```python
from build123d import *

# Parameters (mm, degrees)
SKETCH1_W           = 38
SKETCH1_H           = 41.8
SKETCH1_W_2         = 34.6
SKETCH1_H_2         = 40
BOSS_EXTRUDE1_DEPTH = 100
SKETCH2_W           = 1.7
SKETCH2_H           = 25
BOSS_EXTRUDE2_DEPTH = 13.6
BOSS_EXTRUDE5_DEPTH = 25
SKETCH6_W           = 38
SKETCH6_H           = 41.8
BOSS_EXTRUDE6_DEPTH = 0.6
SKETCH7_W           = 13.3
SKETCH7_H           = 4.4
CUT_EXTRUDE1_DEPTH  = 10
CUT_EXTRUDE2_DEPTH  = 10


with BuildPart() as part:
    # Sketch1 → Boss-Extrude1 (new body)
    with BuildSketch(Plane(origin=(0, 0, 0), x_dir=(1, 0, 0), z_dir=(0, 1, 0))):
        Rectangle(SKETCH1_W, SKETCH1_H)
        Rectangle(SKETCH1_W_2, SKETCH1_H_2, mode=Mode.SUBTRACT)
    extrude(amount=BOSS_EXTRUDE1_DEPTH)

    # Sketch2 → Boss-Extrude2 (add)
    with BuildSketch(Plane(origin=(0, 100, 0), x_dir=(1, 0, 0), z_dir=(0, 1, 0))):
        with Locations((18.15, 0)):
            Rectangle(SKETCH2_W, SKETCH2_H)
        with Locations((-18.15, 0)):
            Rectangle(SKETCH2_W, SKETCH2_H)
    extrude(amount=BOSS_EXTRUDE2_DEPTH)

    # Sketch5 → Boss-Extrude5 (add)
    with BuildSketch(Plane.XY.offset(12.5)):
        Polygon((-15.8, 110), (-17.3, 108.4), (-17.3, 113.6), align=None)
        Polygon((17.3, 108.4), (17.3, 113.6), (15.8, 110), align=None)
    extrude(amount=-BOSS_EXTRUDE5_DEPTH)

    # Sketch6 → Boss-Extrude6 (add)
    with BuildSketch(Plane.XZ):
        Rectangle(SKETCH6_W, SKETCH6_H)
    extrude(amount=BOSS_EXTRUDE6_DEPTH)

    # Sketch7 → Cut-Extrude1 (cut)
    with BuildSketch(Plane(origin=(0, 0, -20.9), x_dir=(-1, 0, 0), z_dir=(0, 0, -1))):
        with Locations((-10.65, 97.8)):
            Rectangle(SKETCH7_W, SKETCH7_H)
    extrude(amount=-CUT_EXTRUDE1_DEPTH, mode=Mode.SUBTRACT)

    # Sketch8 → Cut-Extrude2 (cut)
    with BuildSketch(Plane(origin=(19, 0, 0), x_dir=(0, 0, -1), z_dir=(1, 0, 0))):
        with BuildLine():
            Line((-1, 9.4), (-1, 90))
            ThreePointArc((-1, 90), (0, 91), (1, 90))
            Line((1, 90), (1, 9.4))
            ThreePointArc((1, 9.4), (0, 8.4), (-1, 9.4))
        make_face()
    extrude(amount=-CUT_EXTRUDE2_DEPTH, mode=Mode.SUBTRACT)


solid = part.part
```
Source: CAD feature listing. Evaluate the final solid. Frame: model axes, mm. A direction names the side the tool comes from. Round coordinates to 2 decimals unless told otherwise and drop trailing zeros. Loops run counter-clockwise (first coordinate to the right, second up) from the corner with the lowest first, then second, coordinate; pieces in that order, holes last. Notation, with made-up numbers: M 5.25,18 L 38.25,18 A37 ccw 38.25,56 Z; hole C -19.5,75 d7. An arc over 180 degrees is marked long. Put each result on its own line as item: value.
(1) Section B-B, the plane x = 7. Return loops of the section in (y, z), and give its area (3 significant figures).
Solutions:
outline: M -0.6,-20.9 L 95.6,-20.9 L 95.6,-20 L 0,-20 L 0,20 L 100,20 L 100,20.9 L -0.6,20.9 Z
area: 201 mm²
(2) Access query for faces 1 (the face through (-11.8, 100, -20.5)), 2 (the face through (18, 107, 12.5)), 3 (the face through (0, 49, 20)). Directions: +Z, -Z, +X, -X, +Y, -Y. A direction counts if a zero-diameter tool reaches every point of the face in a straight line with its end or side. Return the directions, or none.
Solutions:
face 1: -Z, +X, -X, +Y
face 2: +Z, +X, -X, +Y
face 3: +Y
(3) Ray query, line 1 (X direction, y = 54.5, z = -5); line 2 (Z direction, x = 2, y = 79); line 3 (Y direction, x = -7, z = 11.5). Return the intervals inside material, ascending. Write a range as [from, to].
Solutions:
line 1: [-19, -17.3], [17.3, 19]
line 2: [-20.9, -20], [20, 20.9]
line 3: [-0.6, 0]
(4) Section A-A, the plane y = 101.5. Return loops of the section in (x, z).
Solutions:
outline: M -19,-12.5 L -17.3,-12.5 L -17.3,12.5 L -19,12.5 Z; M 17.3,-12.5 L 19,-12.5 L 19,12.5 L 17.3,12.5 Z
(5) Pull-direction query (X, two-part tool) for faces 4 (the face through (-19, 57, 0)), 5 (the face through (-18, 107, 12.5)), 6 (the face through (0, 0, 0)); classes: released by +X, released by -X, zero draft, split by the parting line, or undercut.
Solutions:
face 4: released by -X
face 5: zero draft
face 6: undercut
(6) Section D-D, the plane y = 76. Return loops of the section in (x, z).
Solutions:
outline: M -19,-20.9 L 19,-20.9 L 19,-1 L 17.3,-1 L 17.3,-20 L -17.3,-20 L -17.3,20 L 17.3,20 L 17.3,1 L 19,1 L 19,20.9 L -19,20.9 Z
(7) Section C-C, the plane z = 7. Return loops of the section in (x, y), and give its area (3 significant figures).
Solutions:
outline: M -19,-0.6 L 19,-0.6 L 19,113.6 L 17.3,113.6 L 15.8,110 L 17.3,108.4 L 17.3,0 L -17.3,0 L -17.3,108.4 L -15.8,110 L -17.3,113.6 L -19,113.6 Z
area: 417 mm²
(8) First-contact query: pin 1 (1 mm diameter, centred on x = -18, y = 106, fed in from -Z); pin 2 (2.5 mm diameter, centred on x = -4, z = 16.5, fed in from +Y); pin 3 (2.5 mm diameter, centred on x = 17, y = 104.5, fed in from +Z). Flat tips, straight axial feed; report the tip coordinate or a pass-through.
Solutions:
pin 1: z = -12.5
pin 2: y = 0
pin 3: z = 12.5
